Design review of the part shown in the three views and the two pictorial views. Dimensions are in mm from the part's minimum x, y and z. Coordinates: 2 decimals unless noted, no trailing zeros. Write each loop counter-clockwise with the first axis right and the second up, starting at its lowest first coordinate (ties: lowest second). Pieces come first, ordered by that corner, then holes. Notation, with made-up numbers: (-16.75, 54) -> (6.25, 54) arc R36 ccw to (6.25, 88) -> close; hole circle Ø1 at (85.25, 55.25). An arc over 180 degrees is marked (long way). Write item = value, one per line. Start each with the question number.
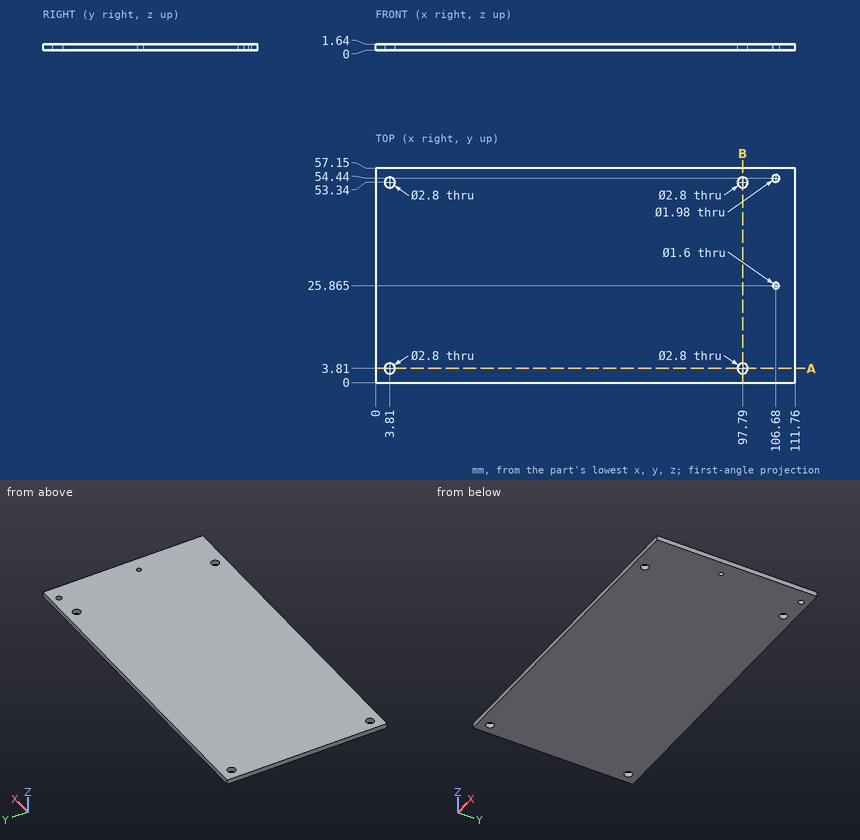
(1) For line 1 (Y direction, x = 3.81, z = 0.7); line 2 (Y direction, x = 106.68, z = 1.2) (3 decimals), list the stretches that pass through material, from the lowest coordinate up.
(2) Take a section at B-B, the plane x = 97.79. State the section outline as (y, z) points, then the cut area to 3 significant figures.
(3) Take a section at A-A, the plane y = 3.81. State the section outline as (x, z) points, then the cut area to 3 significant figures.
(4) For pin 1 Ø1.2 at (x, y) = (106.68, 54.44) entering from +Z, flat-tipped, find the tip position at first contact; note if it passes through.
Report:
q1.line_1 = 0 to 2.41, 5.21 to 51.94, 54.74 to 57.15
q1.line_2 = 0 to 25.065, 26.665 to 53.45, 55.43 to 57.15
q2.outline = (0, 0) -> (2.41, 0) -> (2.41, 1.64) -> (0, 1.64) -> close; (5.21, 0) -> (51.94, 0) -> (51.94, 1.64) -> (5.21, 1.64) -> close; (54.74, 0) -> (57.15, 0) -> (57.15, 1.64) -> (54.74, 1.64) -> close
q2.area = 84.5 mm2
q3.outline = (0, 0) -> (2.41, 0) -> (2.41, 1.64) -> (0, 1.64) -> close; (5.21, 0) -> (96.39, 0) -> (96.39, 1.64) -> (5.21, 1.64) -> close; (99.19, 0) -> (111.76, 0) -> (111.76, 1.64) -> (99.19, 1.64) -> close
q3.area = 174 mm2
q4.pin_1 = through
